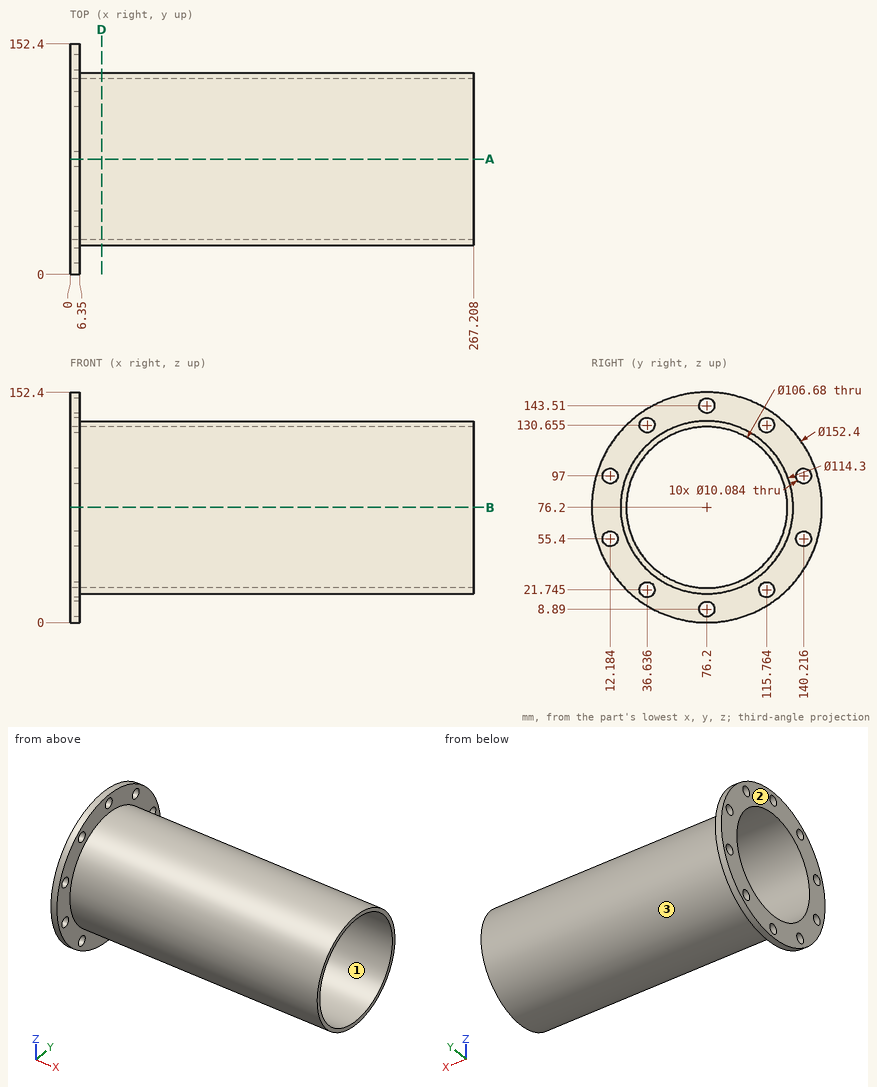
Can you work these out from the drawing? Everything is in mm from the part's minimum corner. Coordinates: 2 decimals unless noted, no trailing zeros. Write each loop counter-clockwise with the first axis right and the second up, starting at its lowest first coordinate (ties: lowest second). Pieces come first, ordered by that corner, then holes. Notation, with made-up numbers: (-4, 78.5) -> (50, 78.5) arc R9 cw to (50, 89.5) -> close; hole circle Ø4 at (7.5, 44.25). An arc over 180 degrees is marked (long way). Write item = value, one per line.
(1) Imagine slicing it at A-A (y = 76.2). Please give me the cut outline in (x, z).
Verdict:
outline = (0, 0) -> (6.35, 0) -> (6.35, 3.85) -> (0, 3.85) -> close; (0, 13.93) -> (6.35, 13.93) -> (6.35, 19.05) -> (267.21, 19.05) -> (267.21, 22.86) -> (0, 22.86) -> close; (0, 129.54) -> (267.21, 129.54) -> (267.21, 133.35) -> (6.35, 133.35) -> (6.35, 138.47) -> (0, 138.47) -> close; (0, 148.55) -> (6.35, 148.55) -> (6.35, 152.4) -> (0, 152.4) -> close
(2) Imagine slicing it at D-D (x = 21). Please give me the cut outline in (y, z).
Verdict:
outline = circle Ø114.3 at (76.2, 76.2); hole circle Ø106.68 at (76.2, 76.2)
(3) For pin 1 (6 mm diameter, centred on x = 33, y = 51, fed in from +Z); pin 2 (3 mm diameter, centred on x = 134.5, z = 42.5, fed in from -Y) (1 decimal); pin 3 (13 mm diameter, centred on y = 36.64, z = 21.75, fed in from +X), each with a flat end and sliding along its axis, tell me the tip position at first contact or that it passes through.
Verdict:
pin_1 = 128.86
pin_2 = 29
pin_3 = 6.35
(4) Imagine slicing it at B-B (z = 76.2). Please give me the cut outline in (x, y), and give its area (3 significant figures).
Verdict:
outline = (0, 0) -> (6.35, 0) -> (6.35, 19.05) -> (267.21, 19.05) -> (267.21, 22.86) -> (0, 22.86) -> close; (0, 129.54) -> (267.21, 129.54) -> (267.21, 133.35) -> (6.35, 133.35) -> (6.35, 152.4) -> (0, 152.4) -> close
area = 2,280 mm^2
(5) Thinking about a two-plate mould opening in Y: for the marked faces 1, 2 and 3, which applies, +Y half, -Y half, draft (parallel to the pull), parting line (faces both ways), or undercut?
Verdict:
face_1 = undercut
face_2 = draft
face_3 = parting line
(6) If I drill on probe 1 along X at (y, z) = (98, 8); probe 2 along Y at (x, z) = (94.5, 85); probe 3 along Z at (x, y) = (74, 117), over which ranges is the centre line in solid material (lowest first)?
Verdict:
probe_1 = 0 to 6.35
probe_2 = 19.73 to 23.59, 128.81 to 132.67
probe_3 = 36.18 to 41.84, 110.56 to 116.22
